Geometry: final body of the model. Coordinates: model frame, mm. Round coordinates to 2 decimals unless told otherwise and drop trailing zeros. Order: outer loops, then holes, each group sorted by start corner. A loop starts at its lowest first (then second) coordinate and runs counter-clockwise, first axis right, second up. Notation, with made-up numbers: (59, 27.5) - (89, 27.5) arc R13 cw to (89, 49.5) - close; hole circle Ø1 at (-36.5, 39). An arc over 180 degrees is marked (long way). Put each result on its own line as item: value. Start each with the question number.
(1) Section D-D (y = 77.5). Output: boundary loops of the cut face in (x, z).
(2) Material intervals for L1, parallel to X at y = 15, z = 1.9; L2, parallel to Y at x = -77, z = 1.5; L3, parallel to Y at x = 77, z = 0.6, sorted ascending. Write a range as [from, to].
(3) Pin query (flat end, axial travel): P1, Ø7, axis at x = 77, y = 13, coming from the +Z side. Return the tip coordinate at first contact, or that it passes through.
(4) Section B-B (x = 77). Output: boundary loops of the cut face in (y, z).
(5) Pull-direction query (X, two-part tool) for faces 1 (the face through (2, 40, 0)), 2 (the face through (-83, 13, 1)), 3 (the face through (-2.1, 75.35, 0.99)); classes: released by +X, released by -X, zero draft, split by the parting line, or undercut.
(6) Section A-A (y = 13). Output: boundary loops of the cut face in (x, z), and give its area (3 significant figures).
(7) Section C-C (z = 1.6). Output: boundary loops of the cut face in (x, y), and give its area (3 significant figures).
from build123d import *

# Parameters (mm, degrees)
SALIENTE_EXTRUIR1_DEPTH = 2
CROQUIS2_R              = 6
CORTAR_EXTRUIR1_DEPTH   = 181.288657436


with BuildPart() as part:
    # Croquis1 → Saliente-Extruir1 (new body)
    with BuildSketch(Plane.XY):
        Polygon((150, 0), (-150, 0), (-150, 100), (150, 50), align=None)
    extrude(amount=SALIENTE_EXTRUIR1_DEPTH)

    # Croquis2 → Cortar-Extruir1 (cut, through all)
    with BuildSketch(Plane.XY.offset(2)):
        with Locations((-77, 13)):
            Circle(CROQUIS2_R)
        with Locations((77, 13)):
            Circle(CROQUIS2_R)
    extrude(amount=-CORTAR_EXTRUIR1_DEPTH, mode=Mode.SUBTRACT)


solid = part.part
Checks:
1. outline: (-150, 0) - (-15, 0) - (-15, 2) - (-150, 2) - close
2. L1: x = [-150, -82.66], [-71.34, 71.34], [82.66, 150]
2. L2: y = [0, 7], [19, 87.83]
2. L3: y = [0, 7], [19, 62.17]
3. P1: passes through
4. outline: (0, 0) - (7, 0) - (7, 2) - (0, 2) - close; (19, 0) - (62.17, 0) - (62.17, 2) - (19, 2) - close
5. face 1: zero draft
5. face 2: undercut
5. face 3: released by +X
6. outline: (-150, 0) - (-83, 0) - (-83, 2) - (-150, 2) - close; (-71, 0) - (71, 0) - (71, 2) - (-71, 2) - close; (83, 0) - (150, 0) - (150, 2) - (83, 2) - close
6. area: 552 mm²
7. outline: (-150, 0) - (150, 0) - (150, 50) - (-150, 100) - close; hole circle Ø12 at (-77, 13); hole circle Ø12 at (77, 13)
7. area: 22,300 mm²
